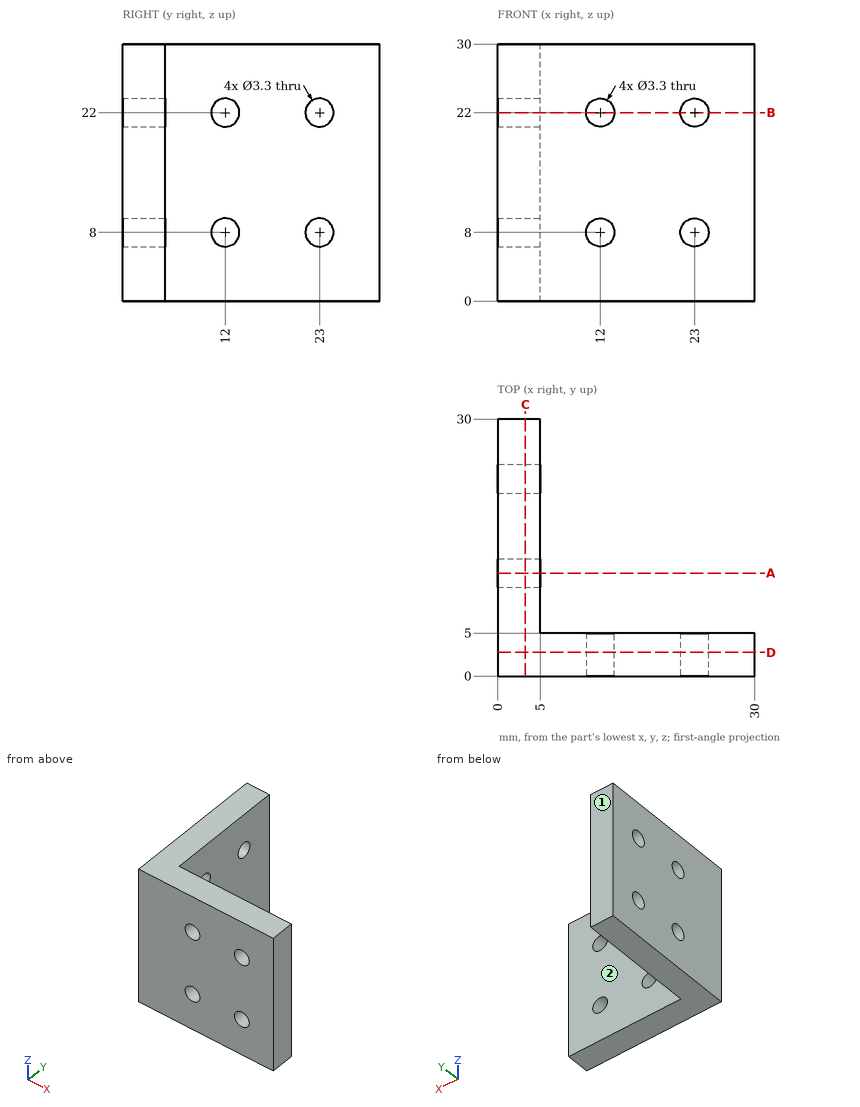
The figure shows three views and two pictorial views of one solid part (mm, origin at its lowest corner). Answer the questions. A direction names the side the tool comes from. Give positions to 0.01 mm unless a question says otherwise; leave off trailing zeros. Order: outer loops, then holes, each group sorted by start corner. A loop starts at its lowest first (then second) coordinate and runs counter-clockwise, first axis right, second up. Notation, with made-up numbers: (63.5, 39.25) - (86.5, 39.25) arc R23 cw to (86.5, 58.25) - close; hole circle Ø7 at (-8, 56.25). An arc over 180 degrees is marked (long way). Answer as CSV lines item,"result".
Q1. Each of these flat-tipped pins is pushed along its axis until it touches: pin 1 Ø4 at (x, z) = (23, 22) entering from -Y; pin 2 Ø4 at (y, z) = (12, 8) entering from +X; pin 3 Ø4 at (x, z) = (9.5, 19.5) entering from +Y. Where does it stop, or does it pass through?
Answer key:
pin 1,"stops at y = 0"
pin 2,"stops at x = 5"
pin 3,"stops at y = 5"
Q2. A cutting plane is placed at A-A, the plane y = 12. Determine the outline of the cut face in (x, z).
Answer key:
outline,"(0, 0) - (5, 0) - (5, 6.35) - (0, 6.35) - close; (0, 9.65) - (5, 9.65) - (5, 20.35) - (0, 20.35) - close; (0, 23.65) - (5, 23.65) - (5, 30) - (0, 30) - close"
Q3. A cutting plane is placed at B-B, the plane z = 22. Determine the outline of the cut face in (x, y).
Answer key:
outline,"(0, 0) - (10.35, 0) - (10.35, 5) - (5, 5) - (5, 10.35) - (0, 10.35) - close; (0, 13.65) - (5, 13.65) - (5, 21.35) - (0, 21.35) - close; (0, 24.65) - (5, 24.65) - (5, 30) - (0, 30) - close; (13.65, 0) - (21.35, 0) - (21.35, 5) - (13.65, 5) - close; (24.65, 0) - (30, 0) - (30, 5) - (24.65, 5) - close"
Q4. Straight lines are drawn through the part: L1, parallel to Z at x = 2, y = 12; L2, parallel to Z at x = 2, y = 23.75; L3, parallel to Y at x = 15.25, z = 17. For each, find the intervals that lie inside material, in ascending order.
Answer key:
L1,"z = 0 to 6.35, 9.65 to 20.35, 23.65 to 30"
L2,"z = 0 to 6.53, 9.47 to 20.53, 23.47 to 30"
L3,"y = 0 to 5"
Q5. Which of the six approach directions +Z, -Z, +X, -X, +Y, -Y give full straight-line access (tool end or side, diameter ignored) to the marked faces 1 and 2?
Answer key:
face 1,"+Z, -Z, +X, -X, +Y"
face 2,"+Z, -Z, +X, +Y"
Q6. A cutting plane is placed at C-C, the plane x = 3.25. Determine the outline of the cut face in (y, z).
Answer key:
outline,"(0, 0) - (30, 0) - (30, 30) - (0, 30) - close; hole circle Ø3.3 at (12, 8); hole circle Ø3.3 at (12, 22); hole circle Ø3.3 at (23, 8); hole circle Ø3.3 at (23, 22)"
